Check sheet for the modelled part. Datum: model origin and axes. Units: mm. Face numbers are marked on the shaded views. A direction names the side the tool comes from. Coordinates: 2 decimals unless noted, no trailing zeros. Loops run counter-clockwise (first coordinate to the right, second up) from the corner with the lowest first, then second, coordinate; pieces in that order, holes last. Notation, with made-up numbers: (2, 27.5) -> (54, 27.5) arc R13 cw to (54, 45.5) -> close; hole circle Ø9 at (-5, -40). An arc over 180 degrees is marked (long way). Use one line per item in the form item = value.
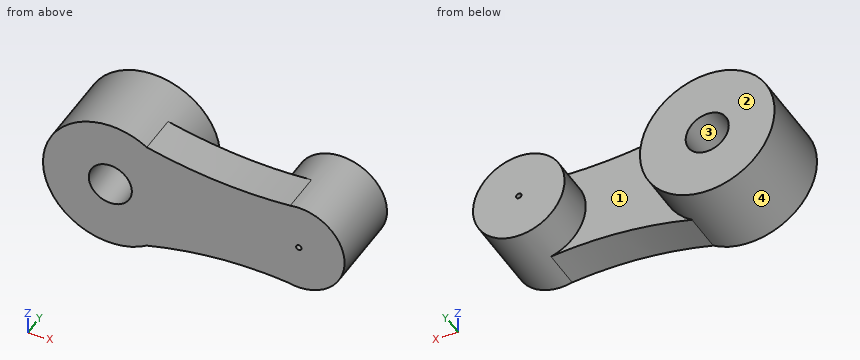
from build123d import *

# Parameters (mm, degrees)
SZKIC1_R                    = 12.5
DODANIE_WYCI_GNI_CIE2_DEPTH = 15
SZKIC3_R                    = 8.5
DODANIE_WYCI_GNI_CIE3_DEPTH = 15
DODANIE_WYCI_GNI_CIE4_DEPTH = 7.5
OTWORY_USTALAJ_CE_8_0MM1_D  = 8
SZKIC7_R                    = 0.5
WYTNIJ_WYCI_GNI_CIE1_DEPTH  = 15


with BuildPart() as part:
    # Szkic1 → Dodanie-wyci_gni_cie2 (new body)
    with BuildSketch(Plane(origin=(0, 0, 0), x_dir=(1, 0, 0), z_dir=(0, 1, 0))):
        with Locations(Location((0, 0, 0), (0, 0, 270))):
            Circle(SZKIC1_R)
    extrude(amount=DODANIE_WYCI_GNI_CIE2_DEPTH)



with BuildPart() as body_2:
    # Szkic3 → Dodanie-wyci_gni_cie3 (new body)
    with BuildSketch(Plane(origin=(0, 0, 0), x_dir=(1, 0, 0), z_dir=(0, 1, 0))):
        with Locations(Location((35, 0, 0), (0, 0, 270))):
            Circle(SZKIC3_R)
    extrude(amount=DODANIE_WYCI_GNI_CIE3_DEPTH)


with BuildPart() as part_1:
    add(part.part)

    add(body_2.part)  # Dodanie-wyci_gni_cie4 merges body 2
    # Szkic4 → Dodanie-wyci_gni_cie4 (add)
    with BuildSketch(Plane(origin=(0, 0, 0), x_dir=(-1, 0, 0), z_dir=(0, -1, 0))):
        with BuildLine():
            ThreePointArc((-6.778939078, 10.502189533), (-12.5, 0), (-6.778939078, -10.502189533))
            add(Edge.make_bspline(
                [(-6.778939078, -10.502189533), (-20.225507154, -7.239536671), (-33.411274741, -8.350206707)],
                knots=[0, 0, 0, 0.631379274, 0.631379274, 0.631379274], degree=2))
            ThreePointArc((-33.411274741, -8.350206707), (-26.503236916, -0.234557237), (-32.953022418, 8.249841379))
            add(Edge.make_bspline(
                [(-6.778939078, 10.502189533), (-20.078070114, 6.877362512), (-32.953022418, 8.249841379)],
                knots=[0, 0, 0, 0.617827196, 0.617827196, 0.617827196], degree=2))
        make_face()
    extrude(amount=-DODANIE_WYCI_GNI_CIE4_DEPTH)

    # Otwory ustalaj_ce _8.0mm1 (through all)
    with Locations(Plane(origin=(0, 15, 0), x_dir=(1, 0, 0), z_dir=(0, 1, 0))):
        with Locations((0, 0)):
            Hole(OTWORY_USTALAJ_CE_8_0MM1_D / 2)

    # Szkic7 → Wytnij-wyci_gni_cie1 (cut)
    with BuildSketch(Plane(origin=(0, 15, 0), x_dir=(1, 0, 0), z_dir=(0, 1, 0))):
        with Locations(Location((35, 0, 0), (0, 0, 270))):
            Circle(SZKIC7_R)
    extrude(amount=-WYTNIJ_WYCI_GNI_CIE1_DEPTH, mode=Mode.SUBTRACT)


solid = part_1.part
(1) Section check B-B, the plane y = 8.5. Record the boundary of the cut face in (x, z).
Established:
outline = circle Ø25 at (0, 0); circle Ø17 at (35, 0); hole circle Ø8 at (0, 0); hole circle Ø1 at (35, 0)
(2) Scan lines: line 1 along Z through (x, y) = (0, 3); line 2 along Z through (x, y) = (35, 11); line 3 along Y through (x, z) = (32, -8). Record each from-to range of solid material in increasing order.
Established:
line_1 = -12.5 to -4, 4 to 12.5
line_2 = -8.5 to -0.5, 0.5 to 8.5
line_3 = 0 to 7.5
(3) Section check A-A, the plane x = 0. Record the boundary of the cut face in (y, z), plus the area to 3 significant figures.
Established:
outline = (0, -12.5) -> (15, -12.5) -> (15, -4) -> (0, -4) -> close; (0, 4) -> (15, 4) -> (15, 12.5) -> (0, 12.5) -> close
area = 255 mm²
(4) Go/stop test with flat-tipped pins: P1, Ø4, axis at x = 29.5, y = 10, coming from the -Z side; P2, Ø6, axis at y = 2, z = 5, coming from the -X side; P3, Ø6, axis at y = 10.5, z = -2, coming from the -X side; P4, Ø1.5, axis at x = 20.5, y = 5.5, coming from the +Z side. Record where each tip stops, or that it passes through.
Established:
P1 = -7.75
P2 = -12.34
P3 = -12.5
P4 = 8.37
(5) Section check C-C, the plane z = 2. Record the boundary of the cut face in (x, y), plus the area to 3 significant figures.
Established:
outline = (-12.34, 0) -> (-3.46, 0) -> (-3.46, 15) -> (-12.34, 15) -> close; (3.46, 0) -> (43.26, 0) -> (43.26, 15) -> (26.74, 15) -> (26.74, 7.5) -> (12.34, 7.5) -> (12.34, 15) -> (3.46, 15) -> close
area = 622 mm²
(6) Tool access check on the marked faces 3 and 4. Record the directions out of +Z, -Z, +X, -X, +Y, -Y that give a thin tool (end or side, any length) a straight path to the whole face; none if there is none.
Established:
face_3 = +Y, -Y
face_4 = +Y
(7) Mould release check, pull along X, two halves, no side actions. Record for the marked faces 1 and 2: +X half, -X half, draft (parallel to the pull), parting line (faces both ways), or undercut.
Established:
face_1 = undercut
face_2 = draft
(8) Section check D-D, the plane z = -5.75. Record the boundary of the cut face in (x, y).
Established:
outline = (-11.1, 0) -> (41.26, 0) -> (41.26, 15) -> (28.74, 15) -> (28.74, 7.5) -> (11.1, 7.5) -> (11.1, 15) -> (-11.1, 15) -> close
